Design review of the part built by this model. Coordinates are the model's own, in mm. A direction names the side the tool comes from. Give positions to 0.01 mm unless a question says otherwise; leave off trailing zeros. Write each loop counter-clockwise with the first axis right and the second up, starting at its lowest first coordinate (ties: lowest second). Pieces come first, ordered by that corner, then holes. Notation, with made-up numbers: (-40, 9) -> (17, 9) arc R10 ccw to (17, 25) -> close; hole circle Ø9 at (35.25, -3). An arc over 180 degrees is marked (long way). Return JSON: item names as keys, results as strings. Group by question number.
from build123d import *

# Parameters (mm, degrees)
SKETCH1_R           = 27.5
SKETCH1_R_2         = 26.5
BOSS_EXTRUDE1_DEPTH = 7
SKETCH2_W           = 14
SKETCH2_H           = 7
BOSS_EXTRUDE2_DEPTH = 3
FILLET1_R           = 1


with BuildPart() as part:
    # Sketch1 → Boss-Extrude1 (new body)
    with BuildSketch(Plane(origin=(0, 0, 0), x_dir=(1, 0, 0), z_dir=(0, 1, 0))):
        with Locations(Location((0, 0, 0), (0, 0, 270))):
            Circle(SKETCH1_R)
        with Locations(Location((0, 0, 0), (0, 0, 270))):
            Circle(SKETCH1_R_2, mode=Mode.SUBTRACT)
    extrude(amount=BOSS_EXTRUDE1_DEPTH)

    # Sketch2 → Boss-Extrude2 (add)
    with BuildSketch(Plane.XY.offset(26.5)):
        with Locations((0, 3.5)):
            Rectangle(SKETCH2_W, SKETCH2_H)
    extrude(amount=BOSS_EXTRUDE2_DEPTH)

    # Fillet1
    fillet1_edges = [part.edges().sort_by_distance(p)[0] for p in [
        (0, 0, 29.5),
        (0, 7, 29.5),
    ]]
    fillet(fillet1_edges, radius=FILLET1_R)


solid = part.part
Q1. Take a section at C-C, the plane y = 4. Give the boundary of the cut face in (x, z), plus the area to 3 significant figures.
Q2. Take a section at A-A, the plane z = 0. Give the boundary of the cut face in (x, y), plus the area to 3 significant figures.
Q3. Insertion check: pin 1 (3 mm diameter, centred on y = 2, z = -5.5, fed in from +X); pin 2 (2.5 mm diameter, centred on y = 4.5, z = 28, fed in from -X); pin 3 (1 mm diameter, centred on x = -18.5, y = 5, fed in from -Z). Each pin has a flat end and moves straight along its axis. Give the tip position at first contact, or say it passes through.
Q4. For L1, parallel to X at y = 4.25, z = 0; L2, parallel to Z at x = -4.5, y = 6.5; L3, parallel to X at y = 5.25, z = 11.5, list the stretches that pass through material, from the lowest coordinate up. Write a range as from..to.
Q5. Take a section at D-D, the plane x = 17. Give the boundary of the cut face in (y, z).
Q6. Take a section at B-B, the plane x = 0. Give the boundary of the cut face in (y, z).
Q7. Mouldability with a two-part tool opening along X and no side actions: class faces 3 (the face through (26.274, 3.451, -3.45)), 4 (the face through (-7, 3, 28)), 5 (the face through (1.11, 3.451, -27.478)) as +X half, -X half, draft (parallel to the pull), parting line (faces both ways), or undercut.
Q8. Tool access review of faces 1 (the face through (-27, 7, 0)), 2 (the face through (7, 3, 28)): name each direction out of +Z, -Z, +X, -X, +Y, -Y from which nothing blocks a thin tool from reaching the whole face with its end or side.
Final values:
{
 "1": {"outline": "(-7, 26.59) arc R27.5 ccw (long way) to (7, 26.59) -> (7, 29.5) -> (-7, 29.5) -> close; hole circle Ø53 at (0, 0)", "area": "202 mm²"},
 "2": {"outline": "(-27.5, 0) -> (-26.5, 0) -> (-26.5, 7) -> (-27.5, 7) -> close; (26.5, 0) -> (27.5, 0) -> (27.5, 7) -> (26.5, 7) -> close", "area": "14.0 mm²"},
 "3": {"pin 1": "stops at x = 27.21", "pin 2": "stops at x = -7", "pin 3": "stops at z = -20.79"},
 "4": {"L1": "x = -27.5..-26.5, 26.5..27.5", "L2": "z = -27.13..-26.12, 26.12..29.37", "L3": "x = -24.98..-23.87, 23.87..24.98"},
 "5": {"outline": "(0, -21.62) -> (7, -21.62) -> (7, -20.33) -> (0, -20.33) -> close; (0, 20.33) -> (7, 20.33) -> (7, 21.62) -> (0, 21.62) -> close"},
 "6": {"outline": "(0, -27.5) -> (7, -27.5) -> (7, -26.5) -> (0, -26.5) -> close; (0, 26.5) -> (7, 26.5) -> (7, 28.5) arc R1 ccw to (6, 29.5) -> (1, 29.5) arc R1 ccw to (0, 28.5) -> close"},
 "7": {"face 3": "undercut", "face 4": "-X half", "face 5": "parting line"},
 "8": {"face 1": "+Z, -Z, +X, -X, +Y", "face 2": "+Z, +X, +Y, -Y"}
}
